Could you check a few things on this drawing? It's one solid part, dimensions in mm from its lowest x, y, z. A direction names the side the tool comes from. Give positions to 0.01 mm unless a question says otherwise; leave off trailing zeros. Loops run counter-clockwise (first coordinate to the right, second up) from the corner with the lowest first, then second, coordinate; pieces in that order, holes last. Notation, with made-up numbers: M -37.5,11 L 18.5,11 A28 ccw 18.5,50 Z; hole C 50.5,0 d7. An arc over 180 degrees is marked long. One line per item, written item: value. Start each with the question number.
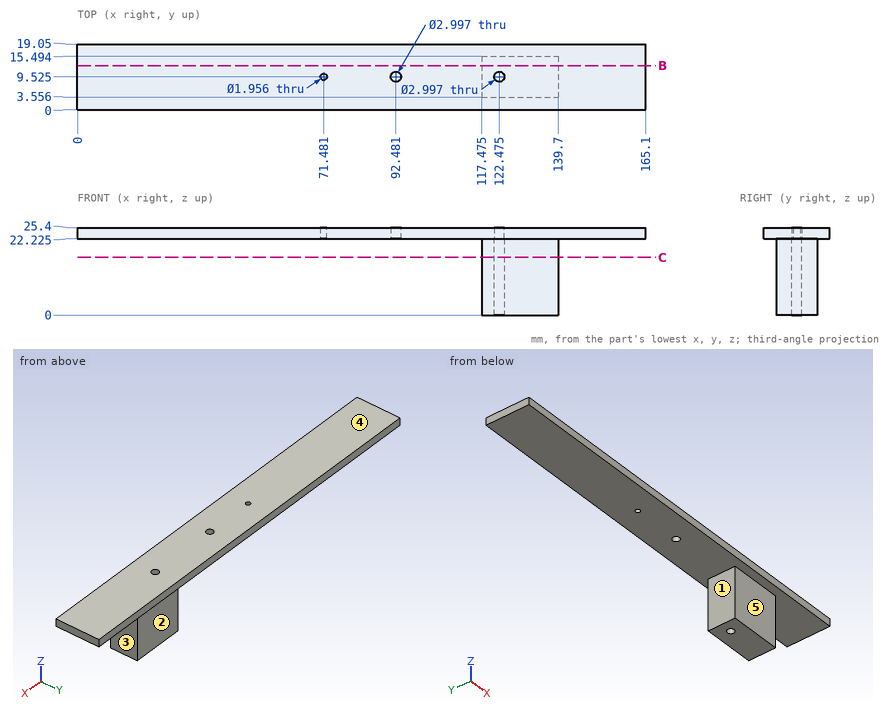
Q1. Which directions (+Z, -Z, +X, -X, +Y, -Y) give clear straight access to the entire face, cutting with the end or side of a thin tool? Please do the marked faces 1, 2, 3, 4 and 5.
Q2. I need wall thicknesses on line 1 along Z through (x, y) = (94, 8.5) (1 decimal); line 2 along X through (y, z) = (14, 14.25) (1 decimal); line 3 along Y through (x, z) = (138.5, 2.5). Which ranges of each line are inside material? Lowest first, please.
Q3. For P1, Ø1.8, axis at x = 122.475, y = 9.525, coming from the +Z side; P2, Ø8, axis at y = 15.5, z = 13, coming from the +X side; P3, Ø1, axis at y = 13.5, z = 15, coming from the -X side (3 decimals); P4, Ø6.5, axis at x = 132, z = 9, coming from the -Y side, each with a flat end and sliding along its axis, tell me the tip position at first contact or that it passes through.
Q4. If we section it at C-C, the plane z = 16.75: Write out the boundary of the cut face in (x, y) (1 decimal), plus the area to 3 significant figures.
Q5. If we section it at B-B, the plane y = 12.75: Write out the boundary of the cut face in (x, z) (1 decimal), plus the area to 3 significant figures.
Response:
1. face 1: -Z, -X, +Y, -Y
1. face 2: -Z, +X, -X, +Y
1. face 3: -Z, +X, +Y, -Y
1. face 4: +Z, +X, -X, +Y, -Y
1. face 5: -Z, +X, -X, -Y
2. line 1: 22.2 to 25.4
2. line 2: 117.5 to 139.7
2. line 3: 3.56 to 15.49
3. P1: through
3. P2: x = 139.7
3. P3: x = 117.475
3. P4: y = 3.56
4. outline: M 117.5,3.6 L 139.7,3.6 L 139.7,15.5 L 117.5,15.5 Z; hole C 122.5,9.5 d3
4. area: 258 mm^2
5. outline: M 0,22.2 L 117.5,22.2 L 117.5,0 L 139.7,0 L 139.7,22.2 L 165.1,22.2 L 165.1,25.4 L 0,25.4 Z
5. area: 1,020 mm^2
